Verification items for the finished model (mm, model axes). A direction names the side the tool comes from. Coordinates: 2 decimals unless noted, no trailing zeros. Order: outer loops, then holes, each group sorted by start corner. A loop starts at its lowest first (then second) coordinate and runs counter-clockwise, first axis right, second up. Notation, with made-up numbers: (68.25, -7.5) -> (75.25, -7.5) arc R15 cw to (75.25, 0.5) -> close; hole circle Ø8 at (76, 15.5). An arc over 180 degrees is marked (long way). Write item = value, one per line. Start each with the question number.
1. Cross-section at A-A on y = 2. Give the number of separate pieces and of enclosed holes in the cut face, plus the area to 3 significant figures.
2. Set-up check for faces 1 (the flat face through (-45, 5, 65)), 2 (the flat face through (-50, 5, -65)), 3 (the cylindrical face through (-18.55, 2.46, -23.38)): record each of +Z, -Z, +X, -X, +Y, -Y from which the full face is reachable in a straight line by a thin tool's end or side.
3. Thickness scan on line 1 along Z through (x, y) = (65, 3.5); line 2 along X through (y, z) = (2.95, -21.5); line 3 along X through (y, z) = (6.15, -21.5) (3 decimals). Record the ranges inside material, lowest first. Write a range as from..to.
4. Release check for a two-part mould opening along X. For faces 4 (the flat face through (90, 4, 1)), 5 (the flat face through (-57, 4, -90)), 6 (the flat face through (20, 5, 22)) record: +X half, -X half, draft (parallel to the pull), parting line (faces both ways), or undercut.
5. Go/stop test with flat-tipped pins: P1, Ø2.5, axis at y = 4.5, z = 67, coming from the -X side; P2, Ø1, axis at y = 2.5, z = 69, coming from the +X side; P3, Ø5, axis at x = -80, z = -65, coming from the +Y side; P4, Ø2.5, axis at x = -80, z = 65, coming from the -Y side. Record where each tip stops, or that it passes through.
6. Cross-section at B-B on x = -30. Record the cut outline in (y, z).
from build123d import *

# Parameters (mm, degrees)
PLATE_DEPTH        = 9
SKETCH3_R          = 1.6
HEX_HOLES_DEPTH    = 128.597021909
SKETCH4_R          = 1.325
LIDAR_HOLES_DEPTH  = 128.597021909
SKETCH5_W          = 100
SKETCH5_H          = 50
SKETCH5_W_2        = 90
CUT_EXTRUDE1_DEPTH = 128.597021909
SKETCH6_R          = 3.5
CUT_EXTRUDE2_DEPTH = 5


with BuildPart() as part:
    # Sketch1 → Plate (new body)
    with BuildSketch(Plane(origin=(0, 0, 0), x_dir=(1, 0, 0), z_dir=(0, 1, 0))):
        with BuildLine():
            Line((-65, -90), (65, -90))
            ThreePointArc((65, -90), (82.67766953, -82.67766953), (90, -65))
            Line((90, -65), (90, 65))
            ThreePointArc((90, 65), (82.67766953, 82.67766953), (65, 90))
            Line((65, 90), (-65, 90))
            ThreePointArc((-65, 90), (-82.67766953, 82.67766953), (-90, 65))
            Line((-90, 65), (-90, -65))
            ThreePointArc((-90, -65), (-82.67766953, -82.67766953), (-65, -90))
        make_face()
    extrude(amount=PLATE_DEPTH)

    # Sketch3 → Hex Holes (cut, through all)
    with BuildSketch(Plane(origin=(0, 9, 0), x_dir=(1, 0, 0), z_dir=(0, 1, 0))):
        with Locations(Location((-65, 80, 0), (0, 0, 270))):
            Circle(SKETCH3_R)
        with Locations(Location((-80, 65, 0), (0, 0, 270))):
            Circle(SKETCH3_R)
        with Locations(Location((80, 65, 0), (0, 0, 270))):
            Circle(SKETCH3_R)
        with Locations(Location((80, -65, 0), (0, 0, 270))):
            Circle(SKETCH3_R)
        with Locations(Location((65, 80, 0), (0, 0, 270))):
            Circle(SKETCH3_R)
        with Locations(Location((65, -80, 0), (0, 0, 270))):
            Circle(SKETCH3_R)
        with Locations(Location((-65, -80, 0), (0, 0, 270))):
            Circle(SKETCH3_R)
        with Locations(Location((-80, -65, 0), (0, 0, 270))):
            Circle(SKETCH3_R)
    extrude(amount=-HEX_HOLES_DEPTH, mode=Mode.SUBTRACT)

    # Sketch4 → LiDAR Holes (cut, through all)
    with BuildSketch(Plane(origin=(0, 9, 0), x_dir=(1, 0, 0), z_dir=(0, 1, 0))):
        with Locations(Location((-21.5, 21.5, 0), (0, 0, 270))):
            Circle(SKETCH4_R)
        with Locations(Location((21.5, 21.5, 0), (0, 0, 270))):
            Circle(SKETCH4_R)
        with Locations(Location((21.5, -21.5, 0), (0, 0, 270))):
            Circle(SKETCH4_R)
        with Locations(Location((-21.5, -21.5, 0), (0, 0, 270))):
            Circle(SKETCH4_R)
    extrude(amount=-LIDAR_HOLES_DEPTH, mode=Mode.SUBTRACT)

    # Sketch5 → Cut-Extrude1 (cut, through all)
    with BuildSketch(Plane(origin=(0, 9, 0), x_dir=(1, 0, 0), z_dir=(0, 1, 0))):
        with Locations((0, 65)):
            Rectangle(SKETCH5_W, SKETCH5_H)
        with Locations((0, -65)):
            Rectangle(SKETCH5_W_2, SKETCH5_H)
    extrude(amount=-CUT_EXTRUDE1_DEPTH, mode=Mode.SUBTRACT)

    # Sketch6 → Cut-Extrude2 (cut)
    with BuildSketch(Plane.XZ):
        with Locations(Location((-21.5, 21.5, 0), (0, 0, 270))):
            Circle(SKETCH6_R)
        with Locations(Location((21.5, 21.5, 0), (0, 0, 270))):
            Circle(SKETCH6_R)
        with Locations(Location((-21.5, -21.5, 0), (0, 0, 270))):
            Circle(SKETCH6_R)
        with Locations(Location((21.5, -21.5, 0), (0, 0, 270))):
            Circle(SKETCH6_R)
    extrude(amount=-CUT_EXTRUDE2_DEPTH, mode=Mode.SUBTRACT)


solid = part.part
Worked out:
q1.separate_pieces = 1
q1.enclosed_holes = 12
q1.area = 22,100 mm²
q2.face_1 = +Z, +Y, -Y
q2.face_2 = -Z, +Y, -Y
q2.face_3 = -Y
q3.line_1 = -90..-81.6, -78.4..78.4, 81.6..90
q3.line_2 = -90..-25, -18..18, 25..90
q3.line_3 = -90..-22.825, -20.175..20.175, 22.825..90
q4.face_4 = +X half
q4.face_5 = draft
q4.face_6 = undercut
q5.P1 = -89.99
q5.P2 = 89.75
q5.P3 = 9
q5.P4 = through
q6.outline = (0, -40) -> (9, -40) -> (9, 40) -> (0, 40) -> close
